Input: part model. Units: mm. Frame: model coordinates. Face numbers are marked on the shaded views. A direction names the side the tool comes from. Coordinates: 2 decimals unless noted, no trailing zeros. Loops run counter-clockwise (first coordinate to the right, second up) from the corner with the lowest first, then second, coordinate; pieces in that order, holes last. Notation, with made-up numbers: (62.25, -20.5) -> (95.25, -20.5) arc R29 cw to (95.25, 7.5) -> close; hole circle Ø7 at (9.5, 73.25). An arc over 180 degrees is marked (long way). Put each result on its own line as item: value. Start each with the question number.
1) Set-up query: the marked faces 1, 2, 3 and 4. Return all of +Z, -Z, +X, -X, +Y, -Y with unobstructed straight access to the full face (end or side cutting, diameter ignored); none if empty.
2) Cut plane A-A (z = 0). Return the cut outline in (x, y).
3) Material intervals for L1, parallel to X at y = -2.05, z = -4.5; L2, parallel to X at y = -2.3, z = 5; L3, parallel to X at y = 0.75, z = 0, sorted ascending.
4) Cut plane B-B (x = -6.5). Return the cut outline in (y, z), plus the area to 3 significant figures.
5) Pull-direction query (Z, two-part tool) for the marked faces 5, 6 and 7; classes: pulls with the +Z half, pulls with the -Z half, needs draft (parallel to the pull), parting line crosses it, or undercut.
6) Cut plane D-D (x = -3). Return the cut outline in (y, z), plus the area to 3 significant figures.
7) Cut plane C-C (y = -2.95). Return the cut outline in (x, z).
8) Contact query for flat-ended pins moving along their axis: P1, Ø1.6, axis at y = -3, z = 5.5, coming from the +X side; P2, Ø1.5, axis at x = 6.5, z = -2.5, coming from the -Y side; P3, Ø0.8, axis at x = -2.5, z = -2.5, coming from the -Y side. Output: stop coordinate, or through.
from build123d import *

# Parameters (mm, degrees)
SKETCH_1_W          = 10
SKETCH_1_H          = 12
SKETCH_1_R          = 3.5
EXTRUDE_1_DEPTH     = 1.7
SKETCH_4_W          = 10
SKETCH_4_H          = 12
EXTRUDE_2_DEPTH     = 3.5
EXTRUDE_START       = -1.7
SKETCH_4_4_W        = 3
SKETCH_4_4_H        = 12
EXTRUDE_3_DEPTH     = 1
CUT_EXTRUDE_START   = 3.5
SKETCH_4_3_W        = 2.4
SKETCH_4_3_H        = 1.9
CUT_EXTRUDE_2_DEPTH = 1.5
CUT_EXTRUDE_START_2 = -5.2
SKETCH_5_R          = 0.3
CUT_EXTRUDE_5_DEPTH = 4
SKETCH_5_6_R        = 0.3
SKETCH_5_6_R_2      = 0.75
CUT_EXTRUDE_6_DEPTH = 12.271202243


with BuildPart() as part:
    # 草图1 → 凸台-拉伸1 (new body)
    with BuildSketch(Plane(origin=(0, 0, 0), x_dir=(1, 0, 0), z_dir=(0, 1, 0))):
        Rectangle(SKETCH_1_W, SKETCH_1_H)
        with Locations(Location((0, 0, 0), (0, 0, 270))):
            Circle(SKETCH_1_R, mode=Mode.SUBTRACT)
    extrude(amount=EXTRUDE_1_DEPTH)

    # 草图4 → 凸台-拉伸2 (add)
    with BuildSketch(Plane.XZ):
        Rectangle(SKETCH_4_W, SKETCH_4_H)
        with BuildLine():
            Line((3.4, 4.1), (3.4, -1.9))
            ThreePointArc((3.4, -1.9), (2.960660172, -2.960660172), (1.9, -3.4))
            Line((1.9, -3.4), (-1.9, -3.4))
            ThreePointArc((-1.9, -3.4), (-2.960660172, -2.960660172), (-3.4, -1.9))
            Line((-3.4, -1.9), (-3.4, 4.1))
            Line((-3.4, 4.1), (3.4, 4.1))
        make_face(mode=Mode.SUBTRACT)
    extrude(amount=EXTRUDE_2_DEPTH)

    # 草图4<4> → 凸台-拉伸3 (add)
    with BuildSketch(Plane.XZ.offset(EXTRUDE_START)):
        with Locations((-6.5, 0)):
            Rectangle(SKETCH_4_4_W, SKETCH_4_4_H)
        with Locations((6.5, 0)):
            Rectangle(SKETCH_4_4_W, SKETCH_4_4_H)
    extrude(amount=EXTRUDE_3_DEPTH)

    # 草图4<3> → 切除-拉伸2 (cut)
    with BuildSketch(Plane.XZ.offset(CUT_EXTRUDE_START)):
        with Locations((-2.2, 5.05)):
            Rectangle(SKETCH_4_3_W, SKETCH_4_3_H)
        with Locations((2.2, 5.05)):
            Rectangle(SKETCH_4_3_W, SKETCH_4_3_H)
        with BuildLine():
            Line((1.3, -6), (1.3, -3.4))
            Line((1.3, -3.4), (0.830662386, -3.4))
            ThreePointArc((0.830662386, -3.4), (0, -3.5), (-0.830662386, -3.4))
            Line((-0.830662386, -3.4), (-1.3, -3.4))
            Line((-1.3, -3.4), (-1.3, -6))
            Line((-1.3, -6), (1.3, -6))
        make_face()
        with BuildLine():
            ThreePointArc((-0.830662386, -3.4), (0, -3.5), (0.830662386, -3.4))
            Line((0.830662386, -3.4), (-0.830662386, -3.4))
        make_face()
    extrude(amount=-CUT_EXTRUDE_2_DEPTH, mode=Mode.SUBTRACT)

    # 草图5 → 切除-拉伸5 (cut)
    with BuildSketch(Plane(origin=(0, 1.7, 0), x_dir=(1, 0, 0), z_dir=(0, 1, 0)).offset(CUT_EXTRUDE_START_2)):
        with Locations(Location((3.5, 4.5, 0), (0, 0, 270))):
            Circle(SKETCH_5_R)
        with Locations(Location((-3.5, 4.5, 0), (0, 0, 270))):
            Circle(SKETCH_5_R)
        with Locations(Location((0, -5.05, 0), (0, 0, 270))):
            Circle(SKETCH_5_R)
    extrude(amount=CUT_EXTRUDE_5_DEPTH, mode=Mode.SUBTRACT)

    # 草图5<6> → 切除-拉伸6 (cut, through all)
    with BuildSketch(Plane(origin=(0, 1.7, 0), x_dir=(1, 0, 0), z_dir=(0, 1, 0))):
        with Locations(Location((3.5, 4.5, 0), (0, 0, 270))):
            Circle(SKETCH_5_6_R)
        with Locations(Location((-3.5, 4.5, 0), (0, 0, 270))):
            Circle(SKETCH_5_6_R)
        with Locations(Location((0, -5.05, 0), (0, 0, 270))):
            Circle(SKETCH_5_6_R)
        with Locations(Location((6.5, 0, 0), (0, 0, 270))):
            Circle(SKETCH_5_6_R_2)
        with Locations(Location((-6.5, 3, 0), (0, 0, 270))):
            Circle(SKETCH_5_6_R_2)
        with Locations(Location((-6.5, -3, 0), (0, 0, 270))):
            Circle(SKETCH_5_6_R_2)
    extrude(amount=-CUT_EXTRUDE_6_DEPTH, mode=Mode.SUBTRACT)


solid = part.part
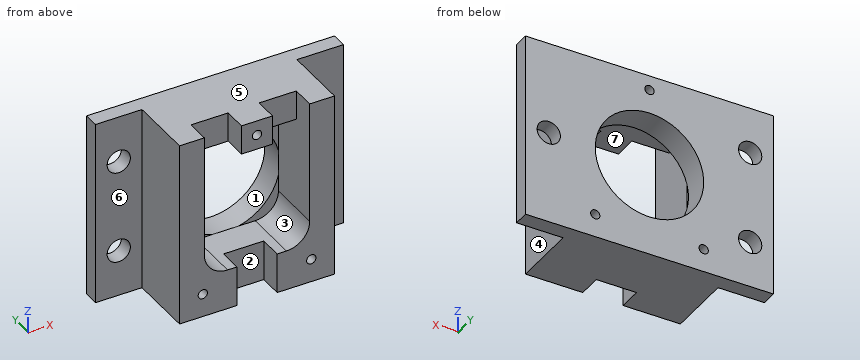
Results found:
1. face 1: +Y
1. face 2: -Z, -Y
1. face 3: -Y
1. face 4: +Z, -Z, +X, -Y
2. outline: (-8, 0.7) -> (-5, 0.7) -> (-5, -3.5) -> (-3.4, -3.5) -> (-3.4, 0) -> (-3.5, 0) -> (-3.5, 1.7) -> (-8, 1.7) -> close; (3.4, -3.5) -> (5, -3.5) -> (5, 0.7) -> (5.75, 0.7) -> (5.75, 1.7) -> (3.5, 1.7) -> (3.5, 0) -> (3.4, 0) -> close; (7.25, 0.7) -> (8, 0.7) -> (8, 1.7) -> (7.25, 1.7) -> close
3. L1: x = -5 to -3.8, -3.2 to -1.3, 1.3 to 3.2, 3.8 to 5
3. L2: x = -5 to -3.4, -1 to -0.3, 0.3 to 1, 3.4 to 5
3. L3: x = -8 to -3.5, 3.5 to 5.75, 7.25 to 8
4. outline: (0.7, -6) -> (1.7, -6) -> (1.7, -3.75) -> (0.7, -3.75) -> close; (0.7, -2.25) -> (1.7, -2.25) -> (1.7, 2.25) -> (0.7, 2.25) -> close; (0.7, 3.75) -> (1.7, 3.75) -> (1.7, 6) -> (0.7, 6) -> close
4. area: 9.00 mm2
5. face 5: pulls with the +Z half
5. face 6: needs draft
5. face 7: undercut
6. outline: (-3.5, -6) -> (1.7, -6) -> (1.7, -1.8) -> (0, -1.8) -> (0, -2.92) -> (-3.5, -2.92) -> close; (-2, 4.1) -> (0, 4.1) -> (0, 1.8) -> (1.7, 1.8) -> (1.7, 6) -> (-2, 6) -> close
6. area: 28.9 mm2
7. outline: (-5, -6) -> (-1.3, -6) -> (-1.3, -3.4) -> (-1.9, -3.4) arc R1.5 cw to (-3.4, -1.9) -> (-3.4, 6) -> (-5, 6) -> close; (-1, 4.1) -> (1, 4.1) -> (1, 6) -> (-1, 6) -> close; (1.3, -6) -> (5, -6) -> (5, 6) -> (3.4, 6) -> (3.4, -1.9) arc R1.5 cw to (1.9, -3.4) -> (1.3, -3.4) -> close; hole circle Ø0.6 at (-3.5, -4.5); hole circle Ø0.6 at (0, 5.05); hole circle Ø0.6 at (3.5, -4.5)
8. P1: stops at x = 5
8. P2: stops at y = 0.7
8. P3: stops at y = 0
